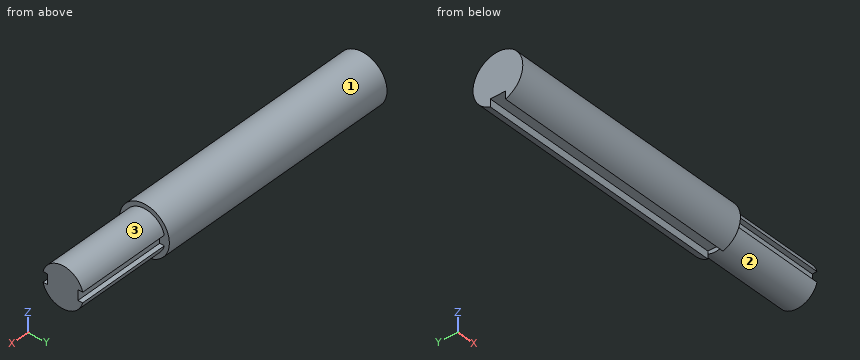
```python
from build123d import *

# Parameters (mm, degrees)
SKETCH1_R           = 6.5
BOSS_EXTRUDE1_DEPTH = 30
SKETCH2_R           = 7.9
BOSS_EXTRUDE2_DEPTH = 80
SKETCH3_W           = 3.2
SKETCH3_H           = 2
CUT_EXTRUDE2_DEPTH  = 30
SKETCH5_W           = 3
SKETCH5_H           = 4.8
CUT_EXTRUDE3_DEPTH  = 80


with BuildPart() as part:
    # Sketch1 → Boss-Extrude1 (new body)
    with BuildSketch(Plane(origin=(0, 0, 0), x_dir=(0, 0, -1), z_dir=(1, 0, 0))):
        Circle(SKETCH1_R)
    extrude(amount=BOSS_EXTRUDE1_DEPTH)

    # Sketch2 → Boss-Extrude2 (add)
    with BuildSketch(Plane.ZY):
        Circle(SKETCH2_R)
    extrude(amount=BOSS_EXTRUDE2_DEPTH)

    # Sketch3 → Cut-Extrude2 (cut)
    with BuildSketch(Plane(origin=(30, 0, 0), x_dir=(0, 0, -1), z_dir=(1, 0, 0))):
        with Locations((0, 5.8)):
            Rectangle(SKETCH3_W, SKETCH3_H)
        with Locations((0, -5.8)):
            Rectangle(SKETCH3_W, SKETCH3_H)
    extrude(amount=-CUT_EXTRUDE2_DEPTH, mode=Mode.SUBTRACT)

    # Sketch5 → Cut-Extrude3 (cut)
    with BuildSketch(Plane.ZY.offset(80)):
        with Locations((-6.626619427, 0)):
            Rectangle(SKETCH5_W, SKETCH5_H)
    extrude(amount=-CUT_EXTRUDE3_DEPTH, mode=Mode.SUBTRACT)


solid = part.part
```
The model under review builds one solid part; all positions refer to its coordinate system, in mm. Face numbers are marked on the shaded views. A direction names the side the tool comes from. Give positions to 0.01 mm unless a question says otherwise; leave off trailing zeros. Order: outer loops, then holes, each group sorted by start corner. A loop starts at its lowest first (then second) coordinate and runs counter-clockwise, first axis right, second up. Notation, with made-up numbers: (-29, 86.25) - (2, 86.25) arc R6 cw to (2, 90.25) - close; hole circle Ø2 at (70, -22.75). An arc over 180 degrees is marked (long way). Use CSV: the item, a comma, the result in double quotes. Start each with the question number.
Q1. To check wall thickness, follow line 1 along Z through (x, y) = (-9.5, 4.5); line 2 along X through (y, z) = (1.75, 7.25). State the ranges of each line that lie inside material, in increasing order. Write a range as [from, to].
Q2. We need section A-A, the plane x = 21. Write out the cut boundary in (y, z).
Q3. Clearance check with flat-ended pins moving along their axes: pin 1 Ø2 at (x, y) = (-21.5, 5) entering from -Z; pin 2 Ø0.8 at (x, y) = (11.5, -5.5) entering from -Z; pin 3 Ø1 at (x, y) = (-62, 2) entering from +Z. State where each tip first meets the part, or that it passes through.
Q4. We need section B-B, the plane z = 0. Write out the cut boundary in (x, y).
Q5. Tool access review of the marked faces 1, 2 and 3: name each direction out of +Z, -Z, +X, -X, +Y, -Y from which nothing blocks a thin tool from reaching the whole face with its end or side.
Outcome:
1,line 1,"z = [-6.49, 6.49]"
1,line 2,"x = [-80, 0]"
2,outline,"(-6.3, -1.6) arc R6.5 ccw to (6.3, -1.6) - (4.8, -1.6) - (4.8, 1.6) - (6.3, 1.6) arc R6.5 ccw to (-6.3, 1.6) - (-4.8, 1.6) - (-4.8, -1.6) - close"
3,pin 1,"stops at z = -6.81"
3,pin 2,"stops at z = -4.03"
3,pin 3,"stops at z = 7.76"
4,outline,"(-80, -7.9) - (0, -7.9) - (0, -4.8) - (30, -4.8) - (30, 4.8) - (0, 4.8) - (0, 7.9) - (-80, 7.9) - close"
5,face 1,"+X, -X"
5,face 2,"-Z, +X"
5,face 3,"+Z, +X"
